The figure shows three views and two pictorial views of one solid part (mm, origin at its lowest corner). Answer the questions. Coordinates: 2 decimals unless noted, no trailing zeros. Write each loop counter-clockwise with the first axis right and the second up, starting at its lowest first coordinate (ties: lowest second). Pieces come first, ordered by that corner, then holes.
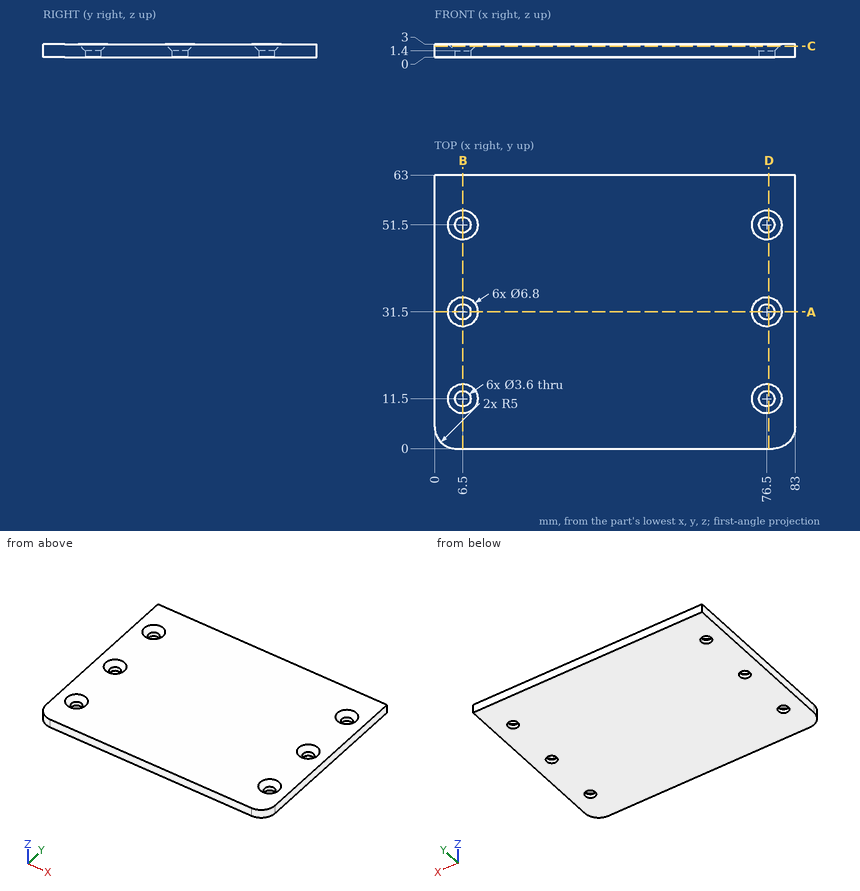
Q1. The part is cut by section B-B, the plane x = 6.5. Write down the section's boundary in (y, z), then the cut area to 3 significant figures.
Answers below:
outline: (0, 0) - (9.7, 0) - (9.7, 1.4) - (8.1, 3) - (0, 3) - close; (13.3, 0) - (29.7, 0) - (29.7, 1.4) - (28.1, 3) - (14.9, 3) - (13.3, 1.4) - close; (33.3, 0) - (49.7, 0) - (49.7, 1.4) - (48.1, 3) - (34.9, 3) - (33.3, 1.4) - close; (53.3, 0) - (63, 0) - (63, 3) - (54.9, 3) - (53.3, 1.4) - close
area: 149 mm2
Q2. The part is cut by section A-A, the plane y = 31.5. Write down the section's boundary in (x, z).
Answers below:
outline: (0, 0) - (4.7, 0) - (4.7, 1.4) - (3.1, 3) - (0, 3) - close; (8.3, 0) - (74.7, 0) - (74.7, 1.4) - (73.1, 3) - (9.9, 3) - (8.3, 1.4) - close; (78.3, 0) - (83, 0) - (83, 3) - (79.9, 3) - (78.3, 1.4) - close
Q3. The part is cut by section D-D, the plane x = 77. State how many separate pieces and enclosed holes the cut face has, then the cut area to 3 significant figures.
Answers below:
separate pieces: 4
enclosed holes: 0
area: 150 mm2
Q4. The part is cut by section C-C, the plane z = 2.5. Write down the section's boundary in (x, y), then the cut area to 3 significant figures.
Answers below:
outline: (0, 5) arc R5 ccw to (5, 0) - (78, 0) arc R5 ccw to (83, 5) - (83, 63) - (0, 63) - close; hole circle Ø5.8 at (6.5, 11.5); hole circle Ø5.8 at (6.5, 31.5); hole circle Ø5.8 at (6.5, 51.5); hole circle Ø5.8 at (76.5, 11.5); hole circle Ø5.8 at (76.5, 31.5); hole circle Ø5.8 at (76.5, 51.5)
area: 5,060 mm2
Q5. Given pin 1 (4 mm diameter, centred on x = 6.5, y = 11.5, fed in from -Z); pin 2 (4.5 mm diameter, centred on x = 76.5, y = 11.5, fed in from +Z); pin 3 (6 mm diameter, centred on x = 6.5, y = 31.5, fed in from +Z), each flat-ended and moving along its own axis, determine where each tip first touches the part or whether it passes through.
Answers below:
pin 1: stops at z = 0
pin 2: stops at z = 1.85
pin 3: stops at z = 2.6
Q6. Find the intervals of material crossed by probe 1 along X at (y, z) = (31.5, 0.95); probe 2 along Y at (x, z) = (76.5, 0.9); probe 3 along X at (y, z) = (30.5, 2.65), in increasing order.
Answers below:
probe 1: x = 0 to 4.7, 8.3 to 74.7, 78.3 to 83
probe 2: y = 0 to 9.7, 13.3 to 29.7, 33.3 to 49.7, 53.3 to 63
probe 3: x = 0 to 3.62, 9.38 to 73.62, 79.38 to 83
